Read the model definition and answer for the solid it produces. Units are mm, in the model's axes. Give positions to 0.01 mm unless a question says otherwise; leave off trailing zeros. Write each loop counter-clockwise with the first axis right and the second up, starting at its lowest first coordinate (ties: lowest second). Pieces come first, ordered by that corner, then holes. Notation, with made-up numbers: (-9, 28) -> (12, 28) arc R14 cw to (12, 32) -> close; hole circle Ø6 at (-3, -30.5). An arc over 180 degrees is marked (long way). Answer as CSV lines item,"result". Start each with the question number.
1. Find the intervals of material crossed by line 1 (X direction, y = -0.05, z = -0.1); line 2 (Y direction, x = 7.5, z = 0.4); line 3 (Y direction, x = 7, z = -0.05), in increasing order.
2. The part is cut by section B-B, the plane y = -0.25. Determine the outline of the cut face in (x, z).
3. The part is cut by section A-A, the plane z = 0.35. Determine the outline of the cut face in (x, y).
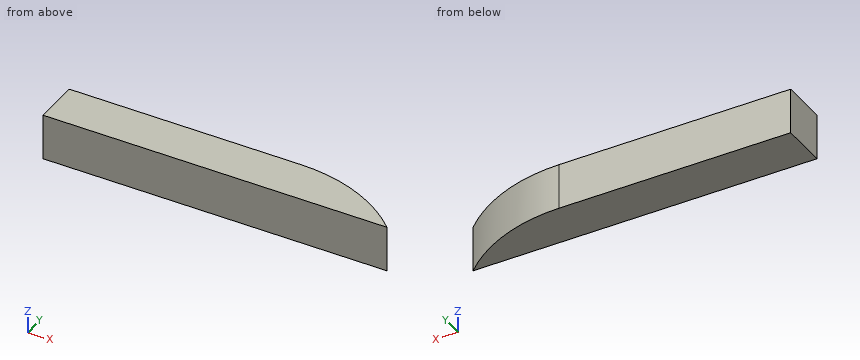
Autodesk Inventor part; units mm, degrees
ref_plane "Work Plane1" through (0, -0.6, 0.6) normal (0, 0, 1) x (1, 0, 0)
ref_plane "YZ Plane" through (0, 0, 0) normal (1, 0, 0) x (0, 1, 0)
ref_plane "XZ Plane" through (0, 0, 0) normal (0, 1, 0) x (-1, 0, 0)
sketch "Sketch1" plane through (0, 0, 0) normal (1, 0, 0) x (0, 1, 0)
  line L0 (-0.6, 0.6) -> (-0.6, -0.6)
  line L1 (-0.6, -0.6) -> (0.6, -0.6)
  line L2 (0.6, -0.6) -> (0.6, 0.6)
  line L3 (0.6, 0.6) -> (-0.6, 0.6)
  line L4 (-0.6, 0.6) -> (0.6, -0.6) construction
  line L5 (-0.6, -0.6) -> (0.6, 0.6) construction
  point P0 (0, 0)
  dimension "d0" = 1.2
  dimension "d1" = 1.2
extrude "Extrusion1" add sketch "Sketch1" along normal blind 9
ref_plane "Work Plane1" through (0, -0.6, 0.6) normal (0, 0, 1) x (1, 0, 0)
sketch "Sketch2" plane through (0, -0.6, 0.6) normal (0, 0, 1) x (1, 0, 0)
  line L0 (9, 0) -> (9, 1.2)
  line L1 (0, 1.2) -> (9, 1.2)
  line L2 (9, 0) -> (9, 1.2)
  line L3 (9, 1.2) -> (7.8, 1.2)
  line L4 (7.8, 1.2) -> (9, 0)
  point P0 (0, 0.6)
  dimension "d5" = 1.2
extrude "Extrusion2" cut sketch "Sketch2" against normal blind 9
fillet "Fillet1" radius 4.2 1 edges at (7.8, 0.6, 0)
properties part number "New_ThinFinger"
Results found:
1,line 1,"x = 0 to 8.3"
1,line 2,"y = -0.6 to 0.35"
1,line 3,"y = -0.6 to 0.49"
2,outline,"(0, -0.6) -> (8.59, -0.6) -> (8.59, 0.6) -> (0, 0.6) -> close"
3,outline,"(0, -0.6) -> (9, -0.6) arc R4.2 ccw to (6.06, 0.6) -> (0, 0.6) -> close"
